Check sheet for the modelled part. Datum: model origin and axes. Units: mm. Round coordinates to 2 decimals unless told otherwise and drop trailing zeros. Order: outer loops, then holes, each group sorted by start corner. A loop starts at its lowest first (then second) coordinate and runs counter-clockwise, first axis right, second up.
Q1. Cross-section at D-D on y = -8. Record the cut outline in (x, z).
Q2. Scan lines: probe 1 along Y at (x, z) = (17, 0.6); probe 2 along Y at (x, z) = (23, 0.9); probe 3 along X at (y, z) = (11, 1.35). Record each from-to range of solid material in increasing order.
Q3. Depth check by flat-ended pin: P1, Ø0.5, axis at x = 15.5, z = 1, coming from the -Y side; P2, Ø0.5, axis at x = -16.5, z = 1, coming from the +Y side; P3, Ø0.5, axis at y = 19.5, z = 0.5, coming from the -X side; P4, Ø4, axis at x = 16, y = -1.5, coming from the -Z side. Enter the tip coordinate at first touch or a pass-through.
Q4. Cross-section at C-C on y = 1. Record the cut outline in (x, z).
Q5. Cross-section at A-A on x = -20. Record the cut outline in (y, z), then the cut area to 3 significant figures.
Q6. Cross-section at B-B on y = 16. Record the cut outline in (x, z), then the cut area to 3 significant figures.
from build123d import *

# Parameters (mm, degrees)
F1_DEPTH = 1.5875
F2_R     = 6.35
F3_R     = 2.54


# Not quite as in the source:
# - a feature names something its author has since deleted; it is built from what else it names


with BuildPart() as f1:
    # F0 (on Top) → F1 (new body)
    with BuildSketch(Plane.XY):
        with BuildLine():
            Line((14.3039512166, 2.778125), (25.2476141741, 2.778125))
            ThreePointArc((25.2476141741, 2.778125), (24.5012506268, 6.6969185243), (23.1505208253, 10.4505208253))
            Line((23.1505208253, 10.4505208253), (10.4505208253, 10.4505208253))
            Line((10.4505208253, 10.4505208253), (10.4505208253, 23.1505208253))
            ThreePointArc((10.4505208253, 23.1505208253), (6.6969185243, 24.5012506268), (2.778125, 25.2476141741))
            Line((2.778125, 25.2476141741), (2.778125, 14.3039512166))
            Line((2.778125, 14.3039512166), (2.778125, 11.0960487834))
            Line((2.778125, 11.0960487834), (0, 9.4920975668))
            Line((0, 9.4920975668), (-2.778125, 11.0960487834))
            Line((-2.778125, 11.0960487834), (-2.778125, 14.3039512166))
            Line((-2.778125, 14.3039512166), (-2.778125, 25.2476141741))
            ThreePointArc((-2.778125, 25.2476141741), (-6.6969185243, 24.5012506268), (-10.4505208253, 23.1505208253))
            Line((-10.4505208253, 23.1505208253), (-10.4505208253, 10.4505208253))
            Line((-10.4505208253, 10.4505208253), (-23.1505208253, 10.4505208253))
            ThreePointArc((-23.1505208253, 10.4505208253), (-24.5012506268, 6.6969185243), (-25.2476141741, 2.778125))
            Line((-25.2476141741, 2.778125), (-14.3039512166, 2.778125))
            Line((-14.3039512166, 2.778125), (-11.0960487834, 2.778125))
            Line((-11.0960487834, 2.778125), (-9.4920975668, 0))
            Line((-9.4920975668, 0), (-11.0960487834, -2.778125))
            Line((-11.0960487834, -2.778125), (-14.3039512166, -2.778125))
            Line((-14.3039512166, -2.778125), (-25.2476141741, -2.778125))
            ThreePointArc((-25.2476141741, -2.778125), (-24.5012506268, -6.6969185243), (-23.1505208253, -10.4505208253))
            Line((-23.1505208253, -10.4505208253), (-10.4505208253, -10.4505208253))
            Line((-10.4505208253, -10.4505208253), (-10.4505208253, -23.1505208253))
            ThreePointArc((-10.4505208253, -23.1505208253), (-6.6969185243, -24.5012506268), (-2.778125, -25.2476141741))
            Line((-2.778125, -25.2476141741), (-2.778125, -14.3039512166))
            Line((-2.778125, -14.3039512166), (-2.778125, -11.0960487834))
            Line((-2.778125, -11.0960487834), (0, -9.4920975668))
            Line((0, -9.4920975668), (2.778125, -11.0960487834))
            Line((2.778125, -11.0960487834), (2.778125, -14.3039512166))
            Line((2.778125, -14.3039512166), (2.778125, -25.2476141741))
            ThreePointArc((2.778125, -25.2476141741), (6.6969185243, -24.5012506268), (10.4505208253, -23.1505208253))
            Line((10.4505208253, -23.1505208253), (10.4505208253, -10.4505208253))
            Line((10.4505208253, -10.4505208253), (23.1505208253, -10.4505208253))
            ThreePointArc((23.1505208253, -10.4505208253), (24.5012506268, -6.6969185243), (25.2476141741, -2.778125))
            Line((25.2476141741, -2.778125), (14.3039512166, -2.778125))
            Line((14.3039512166, -2.778125), (11.0960487834, -2.778125))
            Line((11.0960487834, -2.778125), (9.4920975668, 0))
            Line((9.4920975668, 0), (11.0960487834, 2.778125))
            Line((11.0960487834, 2.778125), (14.3039512166, 2.778125))
        make_face()
    extrude(amount=F1_DEPTH)

    # F2
    f2_edges = [f1.edges().sort_by_distance(p)[0] for p in [
        (-10.450521, -10.450521, 0.79375),
        (10.450521, -10.450521, 0.79375),
        (10.450521, 10.450521, 0.79375),
        (-10.450521, 10.450521, 0.79375),
    ]]
    fillet(f2_edges, radius=F2_R)

    # F3
    f3_edges = [f1.edges().sort_by_distance(p)[0] for p in [
        (2.778125, 25.247614, 0.79375),
        (-2.778125, 25.247614, 0.79375),
        (25.247614, 2.778125, 0.79375),
        (25.247614, -2.778125, 0.79375),
        (2.778125, -25.247614, 0.79375),
        (-2.778125, -25.247614, 0.79375),
        (-25.247614, -2.778125, 0.79375),
        (-25.247614, 2.778125, 0.79375),
        (23.150521, 10.450521, 0.79375),
        (10.450521, -23.150521, 0.79375),
        (-10.450521, -23.150521, 0.79375),
        (-23.150521, -10.450521, 0.79375),
        (-23.150521, 10.450521, 0.79375),
        (-10.450521, 23.150521, 0.79375),
        (10.450521, 23.150521, 0.79375),
        (23.150521, -10.450521, 0.79375),
    ]]
    fillet(f3_edges, radius=F3_R)


solid = f1.part
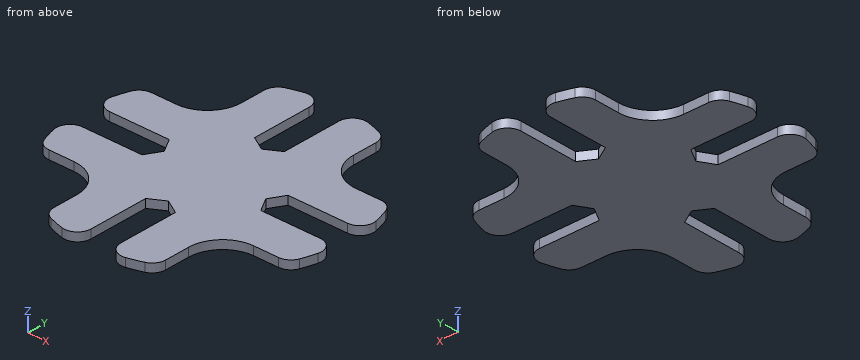
Results found:
1. outline: (-24.11, 0) - (24.11, 0) - (24.11, 1.59) - (-24.11, 1.59) - close
2. probe 1: y = -10.45 to -2.78, 2.78 to 10.45
2. probe 2: y = -9.92 to -2.9, 2.9 to 9.92
2. probe 3: x = -14.22 to -2.61, 2.61 to 14.22
3. P1: stops at y = -10.64
3. P2: stops at y = 10.47
3. P3: stops at x = -10.45
3. P4: stops at z = 0
4. outline: (-10.07, 0) - (10.07, 0) - (10.07, 1.59) - (-10.07, 1.59) - close
5. outline: (-10.45, 0) - (-2.78, 0) - (-2.78, 1.59) - (-10.45, 1.59) - close; (2.78, 0) - (10.45, 0) - (10.45, 1.59) - (2.78, 1.59) - close
5. area: 24.4 mm2
6. outline: (-10.5, 0) - (-2.78, 0) - (-2.78, 1.59) - (-10.5, 1.59) - close; (2.78, 0) - (10.5, 0) - (10.5, 1.59) - (2.78, 1.59) - close
6. area: 24.5 mm2
